```python
from build123d import *

# Parameters (mm, degrees)
EXTRUDE_1_DEPTH          = 1
EXTRUDE_1_DEPTH_BACK     = 1
SKETCH_3_W               = 2
SKETCH_3_H               = 15
EXTRUDE_2_DEPTH          = 1
SKETCH_4_R               = 2
EXTRUDE_3_DEPTH          = 6.5
SKETCH_6_W               = 1
SKETCH_6_H               = 6
CUT_EXTRUDE_1_DEPTH      = 5
EXTRUDE_4_DEPTH          = 3
EXTRUDE_4_DEPTH_BACK     = 3
CUT_EXTRUDE_2_DEPTH      = 5
CUT_EXTRUDE_2_DEPTH_BACK = 5
FILLET_2_R               = 0.1
FILLET_4_R               = 0.1


with BuildPart() as part:
    # Sketch 1 → Extrude 1 (new, two sides: drawn at the far end of the back side and taken through both)
    with BuildSketch(Plane(origin=(0, 0, 0), x_dir=(1, 0, 0), z_dir=(0, 1, 0)).offset(-EXTRUDE_1_DEPTH_BACK)):
        with BuildLine():
            Line((0, -7.5), (0, 7.5))
            Line((0, 7.5), (2, 7.5))
            Line((2, 7.5), (11.380335961, 4.805691692))
            ThreePointArc((11.380335961, 4.805691692), (15, 0), (11.380335961, -4.805691692))
            Line((11.380335961, -4.805691692), (2, -7.5))
            Line((2, -7.5), (0, -7.5))
        make_face()
    extrude(amount=EXTRUDE_1_DEPTH + EXTRUDE_1_DEPTH_BACK)

    # Sketch 3 → Extrude 2 (add)
    with BuildSketch(Plane(origin=(0, 1, 0), x_dir=(1, 0, 0), z_dir=(0, 1, 0))):
        with Locations((1, 0)):
            Rectangle(SKETCH_3_W, SKETCH_3_H)
    extrude_2 = extrude(amount=EXTRUDE_2_DEPTH)

    # Mirror 1: Extrude 2 across plane
    add(extrude_2.mirror(Plane.ZX))

    # Sketch 4 → Extrude 3 (add)
    with BuildSketch(Plane(origin=(0, 1, 0), x_dir=(1, 0, 0), z_dir=(0, 1, 0))):
        with Locations(Location((10, 0, 0), (0, 0, 90))):
            Circle(SKETCH_4_R)
    extrude(amount=EXTRUDE_3_DEPTH)

    # Sketch 5 → Revolve 1 (revolve)
    with BuildSketch(Plane.XY, mode=Mode.PRIVATE) as revolve_1_sk:
        Polygon((8, 7.5), (8, 6.6), (7.9, 6.6), (7.9, 7), align=None)
    revolve(revolve_1_sk.sketch.rotate(Axis((10, 7.5, 0), (0, -1, 0)), 270), axis=Axis((10, 7.5, 0), (0, -1, 0)))

    # Sketch 6 → Cut-Extrude 1 (cut)
    with BuildSketch(Plane(origin=(0, 7.5, 0), x_dir=(1, 0, 0), z_dir=(0, 1, 0))):
        with Locations((10, 0)):
            Rectangle(SKETCH_6_W, SKETCH_6_H)
    extrude(amount=-CUT_EXTRUDE_1_DEPTH, mode=Mode.SUBTRACT)

    # Sketch 7 → Extrude 4 (add, two sides: drawn at the far end of the back side and taken through both)
    with BuildSketch(Plane(origin=(0, 0, 0), x_dir=(1, 0, 0), z_dir=(0, 1, 0)).offset(-EXTRUDE_4_DEPTH_BACK)):
        with BuildLine():
            Line((0, -1.5), (0, 1.5))
            Line((0, 1.5), (-0.677124344, 1.5))
            ThreePointArc((-0.677124344, 1.5), (-1.088161527, 1.780042303), (-1.555590279, 1.95))
            Line((-1.555590279, 1.95), (-2.5, 1.95))
            Line((-2.5, 1.95), (-2.5, -1.95))
            Line((-2.5, -1.95), (-1.555590279, -1.95))
            ThreePointArc((-1.555590279, -1.95), (-1.088161527, -1.780042303), (-0.677124344, -1.5))
            Line((-0.677124344, -1.5), (0, -1.5))
        make_face()
    extrude(amount=EXTRUDE_4_DEPTH + EXTRUDE_4_DEPTH_BACK)

    # Sketch 8 → Cut-Extrude 2 (cut, two sides: drawn at the far end of the back side and taken through both)
    with BuildSketch(Plane.XY.offset(-CUT_EXTRUDE_2_DEPTH_BACK)):
        with BuildLine():
            Line((0, -3), (0, -1.5))
            Line((0, -1.5), (-0.677124344, -1.5))
            ThreePointArc((-0.677124344, -1.5), (-1.088161527, -1.780042303), (-1.555590279, -1.95))
            Line((-1.555590279, -1.95), (-2.5, -1.95))
            Line((-2.5, -1.95), (-2.5, -3))
            Line((-2.5, -3), (0, -3))
        make_face()
        with BuildLine():
            Line((0, 1.5), (-0.677124344, 1.5))
            ThreePointArc((-0.677124344, 1.5), (-1.088161527, 1.780042303), (-1.555590279, 1.95))
            Line((-1.555590279, 1.95), (-2.5, 1.95))
            Line((-2.5, 1.95), (-2.5, 3))
            Line((-2.5, 3), (0, 3))
            Line((0, 3), (0, 1.5))
        make_face()
    extrude(amount=CUT_EXTRUDE_2_DEPTH + CUT_EXTRUDE_2_DEPTH_BACK, mode=Mode.SUBTRACT)

    # Fillet 2
    fillet_2_edges = [part.edges().sort_by_distance(p)[0] for p in [
        (-2.5, 0, 1.95),
        (-2.5, -1.95, 0),
        (-2.5, 0, -1.95),
        (-2.5, 1.95, 0),
        (8, 7.5, 0),
        (12, 7.5, 0),
    ]]
    fillet(fillet_2_edges, radius=FILLET_2_R)

    # Fillet 4
    fillet_4_edges = [part.edges().sort_by_distance(p)[0] for p in [
        (0, 0, 7.5),
        (0, 0, -7.5),
        (0, 2, 0),
        (1, 2, 7.5),
        (2, 2, 0),
        (1, 2, -7.5),
        (0, -2, 0),
        (1, -2, -7.5),
        (2, -2, 0),
        (1, -2, 7.5),
    ]]
    fillet(fillet_4_edges, radius=FILLET_4_R)


solid = part.part
```
CAD build for the part. Positions are in the model's coordinates, mm. A direction names the side the tool comes from. Round coordinates to 2 decimals unless told otherwise and drop trailing zeros. Order: outer loops, then holes, each group sorted by start corner. A loop starts at its lowest first (then second) coordinate and runs counter-clockwise, first axis right, second up.
Q1. Which spindle directions (+Z, -Z, +X, -X, +Y, -Y) get a long thin tool onto all of the face, cutting with end or side? Do faces 1 (the cylindrical face through (-1.09, -0.03, 1.78)), 2 (the cylindrical face through (7.9, 6.8, 0)), 3 (the flat face through (10.5, 5, 0)). Say none if no direction does.
Q2. Slice it at A-A (y = -1.25). Write the cut outline in (x, z), and give its area (3 significant figures).
Q3. Slice it at B-B (x = 10). Write the cut outline in (y, z), and give its area (3 significant figures).
Q4. Drop flat-ended pins along their axis: pin 1 (0.5 mm diameter, centred on x = -0.5, y = 0, fed in from +Z); pin 2 (0.9 mm diameter, centred on x = -2, y = -0.5, fed in from -Z); pin 3 (0.7 mm diameter, centred on x = -0.5, z = -0.5, fed in from -Y). Give the stop position or say it passes through.
Q5. Wall check: L1, parallel to X at y = 6.25, z = 0; L2, parallel to Y at x = 12, z = -2; L3, parallel to Y at x = 10.25, z = -1.5. Give the ranges that are in metal, low to high.
Q6. Slice it at D-D (y = 4). Write the cut outline in (x, z).
Q7. Slice it at C-C (z = 5.5). Write the cut outline in (x, y).
Results below:
1. face 1: +Z, +Y, -Y
1. face 2: -X, +Y
1. face 3: +Z, -Z, +Y
2. outline: (-2.5, -1.85) arc R0.1 ccw to (-2.4, -1.95) - (-1.56, -1.95) arc R2 ccw to (-0.68, -1.5) - (0, -1.5) - (0, -7.4) arc R0.1 ccw to (0.1, -7.5) - (2, -7.5) - (2, 7.5) - (0.1, 7.5) arc R0.1 ccw to (0, 7.4) - (0, 1.5) - (-0.68, 1.5) arc R2 ccw to (-1.56, 1.95) - (-2.4, 1.95) arc R0.1 ccw to (-2.5, 1.85) - close
2. area: 38.8 mm2
3. outline: (-1, -5.2) - (1, -5.2) - (1, -2) - (2.5, -2) - (2.5, 2) - (1, 2) - (1, 5.2) - (-1, 5.2) - close
3. area: 26.8 mm2
4. pin 1: stops at z = 1.56
4. pin 2: stops at z = -1.95
4. pin 3: stops at y = -1.64
5. L1: x = 8 to 9.5, 10.5 to 12
5. L2: y = -1 to 1
5. L3: y = -1 to 2.5
6. outline: (9.5, -1.94) - (9.5, 1.94) arc R2 ccw to start; (10.5, -1.94) arc R2 ccw to (10.5, 1.94) - close
7. outline: (0, -1.9) arc R0.1 ccw to (0.1, -2) - (1.9, -2) arc R0.1 ccw to (2, -1.9) - (2, -1) - (8.96, -1) - (8.96, 1) - (2, 1) - (2, 1.9) arc R0.1 ccw to (1.9, 2) - (0.1, 2) arc R0.1 ccw to (0, 1.9) - close
